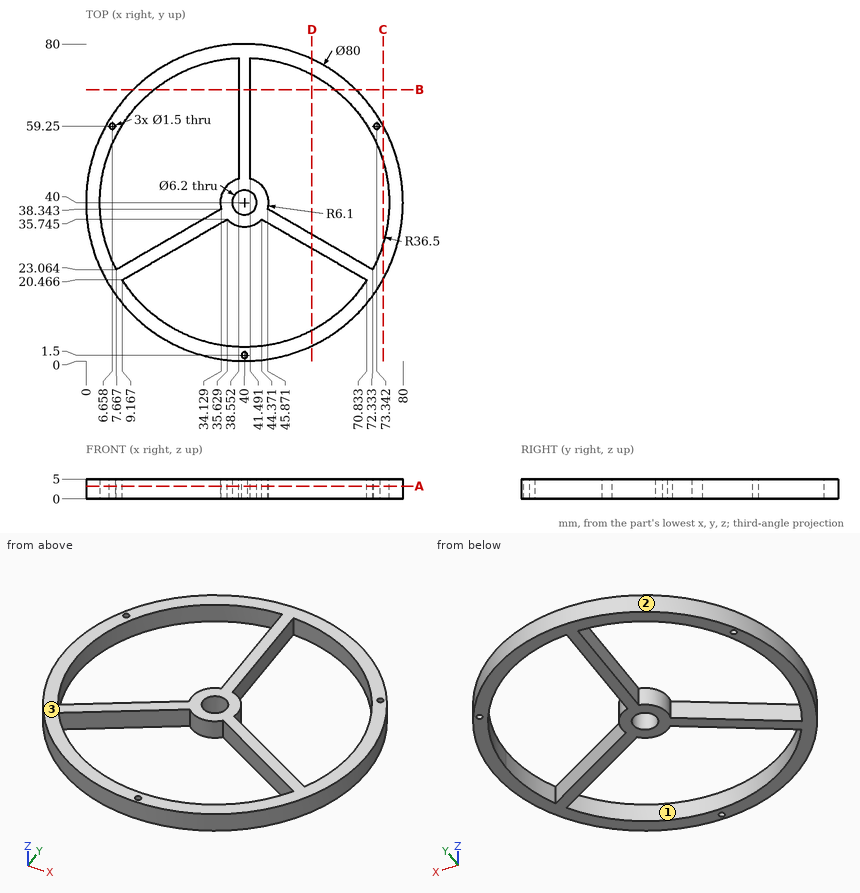
Geometry check sheet. Reference: drawing and pictorial views, mm from the part's lowest x, y, z. Round coordinates to 2 decimals unless told otherwise and drop trailing zeros. Loops run counter-clockwise (first coordinate to the right, second up) from the corner with the lowest first, then second, coordinate; pieces in that order, holes last. Notation, with made-up numbers: M -9.5,70.5 L 4.5,70.5 A10 cw 4.5,78.5 Z; hole C 21,79 d3. An arc over 180 degrees is marked long. Return JSON: item names as keys, results as strings. Group by question number.
(1) Section check A-A, the plane z = 3.2. Give the number of separate pieces and of enclosed holes in the cut face.
(2) Section check B-B, the plane y = 68.5. Enter the section's corners in (x, z).
(3) Mould release check, pull along Y, two halves, no side actions. Record for the marked faces 1, 2 and 3: pulls with the +Y half, pulls with the -Y half, needs draft (parallel to the pull), parting line crosses it, or undercut.
(4) Go/stop test with flat-tipped pins: pin 1 (1.2 mm diameter, centred on x = 6.66, y = 59.25, fed in from +Z); pin 2 (3 mm diameter, centred on y = 17, z = 2, fed in from +X); pin 3 (3 mm diameter, centred on x = 24, z = 4.5, fed in from +Y). Record where each tip stops, or that it passes through.
(5) Scan lines: line 1 along Y through (x, z) = (39.5, 4.6) (1 decimal); line 2 along Y through (x, z) = (33, 2.8) (1 decimal); line 3 along Y through (x, z) = (25.5, 0.9) (1 decimal). Record each from-to range of solid material in increasing order. Write a range as [from, to].
(6) Section check C-C, the plane x = 75. Enter the section's corners in (y, z) (1 decimal).
(7) Section check D-D, the plane x = 57. Enter the section's corners in (y, z).
Data:
{
 "1": {"separate pieces": "1", "enclosed holes": "7"},
 "2": {"outline": "M 11.93,0 L 17.2,0 L 17.2,5 L 11.93,5 Z; M 38.55,0 L 41.49,0 L 41.49,5 L 38.55,5 Z; M 62.8,0 L 68.07,0 L 68.07,5 L 62.8,5 Z"},
 "3": {"face 1": "undercut", "face 2": "parting line crosses it", "face 3": "needs draft"},
 "4": {"pin 1": "through", "pin 2": "x = 73.73", "pin 3": "y = 77.28"},
 "5": {"line 1": "[0, 0.9], [2.1, 3.5], [33.9, 36.9], [43.1, 80]", "line 2": "[0.6, 4.2], [34.2, 37.7], [75.8, 79.4]", "line 3": "[2.7, 6.5], [29.9, 33.4], [73.5, 77.3]"},
 "6": {"outline": "M 20.6,0 L 29.6,0 L 29.6,5 L 20.6,5 Z; M 50.4,0 L 59.4,0 L 59.4,5 L 50.4,5 Z"},
 "7": {"outline": "M 3.79,0 L 7.7,0 L 7.7,5 L 3.79,5 Z; M 28.45,0 L 31.92,0 L 31.92,5 L 28.45,5 Z; M 72.3,0 L 76.21,0 L 76.21,5 L 72.3,5 Z"}
}
